```python
from build123d import *

# Parameters (mm, degrees)
SKETCH_1_W          = 280
SKETCH_1_H          = 90
SKETCH_1_R          = 1.5
SKETCH_1_R_2        = 1.75
SKETCH_1_R_3        = 6
SKETCH_1_R_4        = 8.875
SKETCH_1_W_2        = 15
SKETCH_1_H_2        = 4
SKETCH_1_W_3        = 56
SKETCH_1_H_3        = 30.5
EXTRUDE_1_DEPTH     = 4
SKETCH_2_W          = 20
SKETCH_2_H          = 4
SKETCH_2_W_2        = 4
SKETCH_2_H_2        = 30
SKETCH_2_R          = 1.4
EXTRUDE_2_DEPTH     = 4
SKETCH_3_W          = 5
SKETCH_3_H          = 7.5
CUT_EXTRUDE_1_DEPTH = 153.161098839
FILLET_1_R          = 1.5


with BuildPart() as part:
    # Эскиз1 → Бобышка-Вытянуть1 (new body)
    with BuildSketch(Plane.XY):
        Rectangle(SKETCH_1_W, SKETCH_1_H)
        with Locations((11.25, 6.5)):
            Circle(SKETCH_1_R, mode=Mode.SUBTRACT)
        with Locations((-11.25, 6.5)):
            Circle(SKETCH_1_R, mode=Mode.SUBTRACT)
        with Locations((-11.25, -39.5)):
            Circle(SKETCH_1_R, mode=Mode.SUBTRACT)
        with Locations((11.25, -39.5)):
            Circle(SKETCH_1_R, mode=Mode.SUBTRACT)
        with Locations((113.75, 34.5)):
            Circle(SKETCH_1_R_2, mode=Mode.SUBTRACT)
        with Locations((98.25, 19)):
            Circle(SKETCH_1_R_3, mode=Mode.SUBTRACT)
        with Locations((-98.25, 19)):
            Circle(SKETCH_1_R_4, mode=Mode.SUBTRACT)
        with Locations((113.75, 3.5)):
            Circle(SKETCH_1_R_2, mode=Mode.SUBTRACT)
        with Locations((82.75, 3.5)):
            Circle(SKETCH_1_R_2, mode=Mode.SUBTRACT)
        with Locations((82.75, 34.5)):
            Circle(SKETCH_1_R_2, mode=Mode.SUBTRACT)
        with Locations((-110.75, 19)):
            Circle(SKETCH_1_R_2, mode=Mode.SUBTRACT)
        with Locations((-85.75, 19)):
            Circle(SKETCH_1_R_2, mode=Mode.SUBTRACT)
        with Locations((-127.5, 22.5)):
            Circle(SKETCH_1_R, mode=Mode.SUBTRACT)
        with Locations((-127.5, 0)):
            Circle(SKETCH_1_R, mode=Mode.SUBTRACT)
        with Locations((-127.5, -22.5)):
            Circle(SKETCH_1_R, mode=Mode.SUBTRACT)
        with Locations((-38.5, 22.5)):
            Circle(SKETCH_1_R, mode=Mode.SUBTRACT)
        with Locations((-38.5, 0)):
            Circle(SKETCH_1_R, mode=Mode.SUBTRACT)
        with Locations((-38.5, -22.5)):
            Circle(SKETCH_1_R, mode=Mode.SUBTRACT)
        with Locations((0, -39.5)):
            Rectangle(SKETCH_1_W_2, SKETCH_1_H_2, mode=Mode.SUBTRACT)
        with Locations((0, 6.5)):
            Rectangle(SKETCH_1_W_2, SKETCH_1_H_2, mode=Mode.SUBTRACT)
        with Locations((0, -18)):
            Rectangle(SKETCH_1_W_3, SKETCH_1_H_3, mode=Mode.SUBTRACT)
    extrude(amount=EXTRUDE_1_DEPTH)

    # Эскиз2 → Бобышка-Вытянуть2 (add, through all)
    # profile 1 of 6: a face of its own
    with BuildSketch(Plane.XY.offset(4)):
        with Locations((130, 47)):
            Rectangle(SKETCH_2_W, SKETCH_2_H)
    # profile 2 of 6: a face of its own
    with BuildSketch(Plane.XY.offset(4)):
        with Locations((142, 0)):
            Rectangle(SKETCH_2_W_2, SKETCH_2_H_2)
        with Locations((141.75, 0)):
            Circle(SKETCH_2_R, mode=Mode.SUBTRACT)
    # profile 3 of 6: a face of its own
    with BuildSketch(Plane.XY.offset(4)):
        with Locations((-130, 47)):
            Rectangle(SKETCH_2_W, SKETCH_2_H)
    # profile 4 of 6: a face of its own
    with BuildSketch(Plane.XY.offset(4)):
        with Locations((-142, 0)):
            Rectangle(SKETCH_2_W_2, SKETCH_2_H_2)
        with Locations((-141.75, 0)):
            Circle(SKETCH_2_R, mode=Mode.SUBTRACT)
    # profile 5 of 6: a face of its own
    with BuildSketch(Plane.XY.offset(4)):
        with Locations((67.75, 47)):
            Rectangle(SKETCH_2_W, SKETCH_2_H)
    # profile 6 of 6: a face of its own
    with BuildSketch(Plane.XY.offset(4)):
        with Locations((-67.75, 47)):
            Rectangle(SKETCH_2_W, SKETCH_2_H)
    extrude(amount=-EXTRUDE_2_DEPTH)

    # Эскиз3 → Вырез-Вытянуть1 (cut, through all)
    with BuildSketch(Plane.XY.offset(4)):
        Polygon((14.5, 45), (14.5, 49), (-20.75, 49), (-20.75, 45), (-28.5, 45), (-28.5, 13.75), (-24.75, 10), (10.75, 10), (14.5, 13.75), (14.5, 22.5), (25.5, 22.5), (25.5, 45), align=None)
        Polygon((-97.375, 42), (-97.375, 45), (-100.375, 45), (-100.375, 42), (-101.425, 42), (-101.425, 40), (-100.375, 40), (-100.375, 39), (-97.375, 39), (-97.375, 40), (-96.325, 40), (-96.325, 42), align=None)
        with Locations((137.5, 15.75)):
            Rectangle(SKETCH_3_W, SKETCH_3_H)
        with Locations((-137.5, 15.75)):
            Rectangle(SKETCH_3_W, SKETCH_3_H)
    extrude(amount=-CUT_EXTRUDE_1_DEPTH, mode=Mode.SUBTRACT)

    # Скругление1
    fillet_1_edges = [part.edges().sort_by_distance(p)[0] for p in [
        (140, 12, 2),
        (135, 12, 2),
        (135, 19.5, 2),
        (-135, 12, 2),
        (-140, 12, 2),
        (-135, 19.5, 2),
    ]]
    fillet(fillet_1_edges, radius=FILLET_1_R)


solid = part.part
```
For this review, take the finished solid that the model builds, in its own axes (mm). Round coordinates to 2 decimals unless told otherwise and drop trailing zeros. Write each loop counter-clockwise with the first axis right and the second up, starting at its lowest first coordinate (ties: lowest second). Pieces come first, ordered by that corner, then holes. Notation, with made-up numbers: (22, 67) -> (80, 67) arc R26 ccw to (80, 105) -> close; hole circle Ø4 at (-34, 83.5). An arc over 180 degrees is marked (long way). One line per question, with ' | ' between items. Start each with the question number.
1) Wall thickness on line 1 along Y through (x, z) = (-38.5, 2.35); line 2 along Y through (x, z) = (5.5, 3.3); line 3 along Y through (x, z) = (82.75, 2): over which ranges is each line inside the solid? List them lowest first.
2) Add section B-B (x = 4). Write out the cut boundary in (y, z), and give its area (3 significant figures).
3) Add section C-C (z = 2.9). Count the separate pieces of the cut face and the enclosed holes in it, and give its area (3 significant figures).
4) Add section D-D (x = -93). Write out the cut boundary in (y, z).
5) Mouldability with a two-part tool opening along X and no side actions: class faces 1 (the cylindrical face through (-93.479, 26.483, 1.972)), 2 (the cylindrical face through (92.256, 19.264, 1.972)), 3 (the flat face through (-2, 3, 4)) as +X half, -X half, draft (parallel to the pull), parting line (faces both ways), or undercut.
6) For pin 1 Ø1.2 at (y, z) = (18, 2.5) entering from -X; pin 2 Ø1.2 at (y, z) = (-38.5, 2.5) entering from +X; pin 3 Ø2 at (x, z) = (-4.5, 1) entering from +Y; pin 4 Ø2.5 at (x, y) = (-127.5, 22.5) entering from +Z, all flat-tipped, find the tip position at first contact; note any pin that passes through.
7) Add section A-A (x = 98.25). Write out the cut boundary in (y, z), and give its area (3 significant figures).
Reported:
1) line 1: y = -45 to -24, -21 to -1.5, 1.5 to 21, 24 to 45 | line 2: y = -45 to -41.5, -37.5 to -33.25, -2.75 to 4.5, 8.5 to 10 | line 3: y = -45 to 1.75, 5.25 to 32.75, 36.25 to 45
2) outline: (-45, 0) -> (-41.5, 0) -> (-41.5, 4) -> (-45, 4) -> close; (-37.5, 0) -> (-33.25, 0) -> (-33.25, 4) -> (-37.5, 4) -> close; (-2.75, 0) -> (4.5, 0) -> (4.5, 4) -> (-2.75, 4) -> close; (8.5, 0) -> (10, 0) -> (10, 4) -> (8.5, 4) -> close | area: 66.0 mm²
3) separate pieces: 1 | enclosed holes: 23 | area: 21,600 mm²
4) outline: (-45, 0) -> (11.84, 0) -> (11.84, 4) -> (-45, 4) -> close; (26.16, 0) -> (45, 0) -> (45, 4) -> (26.16, 4) -> close
5) face 1: undercut | face 2: undercut | face 3: draft
6) pin 1: stops at x = -135.13 | pin 2: stops at x = 140 | pin 3: stops at y = 10 | pin 4: passes through
7) outline: (-45, 0) -> (13, 0) -> (13, 4) -> (-45, 4) -> close; (25, 0) -> (45, 0) -> (45, 4) -> (25, 4) -> close | area: 312 mm²
